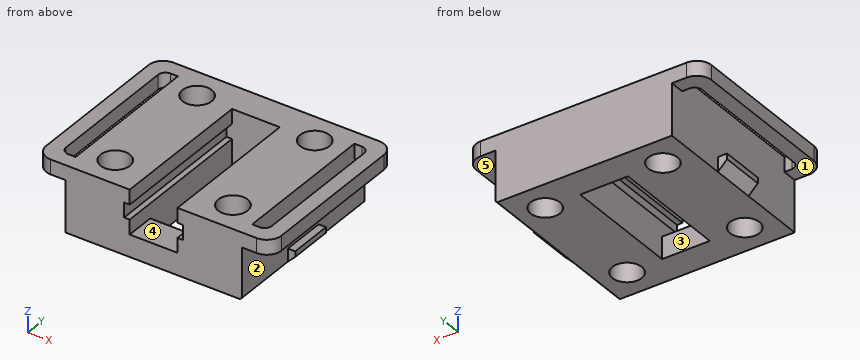
```python
from build123d import *

# Parameters (mm, degrees)
F0_W      = 24
F0_H      = 24
F0_R      = 2
F1_DEPTH  = 9
F3_START  = 7
F2_W      = 32
F2_H      = 24
F2_R      = 2
F2_W_2    = 2
F2_H_2    = 20
F3_DEPTH  = 2
F4_W      = 8
F4_H      = 6
F5_DEPTH  = 12
F6_DEPTH  = 8
F7_W      = 0.75
F7_H      = 2
F8_DEPTH  = 12
F9_W      = 1.25
F9_H      = 6
F10_DEPTH = 2
F11_SIZE  = 1.25
F12_W     = 6.5
F12_H     = 16
F13_DEPTH = 3
F14_R     = 2
F15_R     = 1


with BuildPart() as f1:
    # F0 (on Top) → F1 (new body)
    with BuildSketch(Plane.XY):
        Rectangle(F0_W, F0_H)
        with Locations((-8, -8)):
            Circle(F0_R, mode=Mode.SUBTRACT)
        with Locations((8, -8)):
            Circle(F0_R, mode=Mode.SUBTRACT)
        with Locations((-8, 8)):
            Circle(F0_R, mode=Mode.SUBTRACT)
        with Locations((8, 8)):
            Circle(F0_R, mode=Mode.SUBTRACT)
    extrude(amount=F1_DEPTH)

    # F2 (on Top) → F3 (join)
    with BuildSketch(Plane.XY.offset(F3_START)):
        Rectangle(F2_W, F2_H)
        with Locations((-8, -8)):
            Circle(F2_R, mode=Mode.SUBTRACT)
        with Locations((8, -8)):
            Circle(F2_R, mode=Mode.SUBTRACT)
        with Locations((-13, 0)):
            Rectangle(F2_W_2, F2_H_2, mode=Mode.SUBTRACT)
        with Locations((-8, 8)):
            Circle(F2_R, mode=Mode.SUBTRACT)
        with Locations((13, 0)):
            Rectangle(F2_W_2, F2_H_2, mode=Mode.SUBTRACT)
        with Locations((8, 8)):
            Circle(F2_R, mode=Mode.SUBTRACT)
    extrude(amount=F3_DEPTH)

    # F4 (on Front) → F5 (cut)
    with BuildSketch(Plane.XZ):
        with Locations((0, 6)):
            Rectangle(F4_W, F4_H)
    extrude(amount=F5_DEPTH, mode=Mode.SUBTRACT)

    # F4 (on Front) → F6 (cut)
    with BuildSketch(Plane.XZ):
        with Locations((0, 6)):
            Rectangle(F4_W, F4_H)
    extrude(amount=-F6_DEPTH, mode=Mode.SUBTRACT)

    # F7 (on Front) → F8 (join, symmetric)
    with BuildSketch(Plane.XZ):
        with Locations((-3.625, 8)):
            Rectangle(F7_W, F7_H)
        with Locations((3.625, 8)):
            Rectangle(F7_W, F7_H)
        with Locations((3.625, 4)):
            Rectangle(F7_W, F7_H)
        with Locations((-3.625, 4)):
            Rectangle(F7_W, F7_H)
    extrude(amount=F8_DEPTH, both=True)

    # F9 (on Top) → F10 (join)
    with BuildSketch(Plane.XY):
        with Locations((-12.625, 0)):
            Rectangle(F9_W, F9_H)
        with Locations((12.375, 0)):
            Rectangle(F9_W, F9_H)
    extrude(amount=F10_DEPTH)

    # F11
    f11_edges = [f1.edges().sort_by_distance(p)[0] for p in [
        (13, 0, 0),
        (-13.25, 0, 0),
    ]]
    chamfer(f11_edges, length=F11_SIZE)

    # F12 (on Top) → F13 (cut)
    with BuildSketch(Plane.XY):
        Rectangle(F12_W, F12_H)
    extrude(amount=F13_DEPTH, mode=Mode.SUBTRACT)

    # F14
    f14_edges = [f1.edges().sort_by_distance(p)[0] for p in [
        (16, -12, 8),
        (16, 12, 8),
        (-16, -12, 8),
        (-16, 12, 8),
    ]]
    fillet(f14_edges, radius=F14_R)

    # F15
    f15_edges = [f1.edges().sort_by_distance(p)[0] for p in [
        (-14, 10, 8),
        (-14, -10, 8),
        (14, 10, 8),
        (14, -10, 8),
    ]]
    fillet(f15_edges, radius=F15_R)


solid = f1.part
```
Check sheet for the modelled part. Datum: model origin and axes. Units: mm. Face numbers are marked on the shaded views. A direction names the side the tool comes from. Give positions to 0.01 mm unless a question says otherwise; leave off trailing zeros. Order: outer loops, then holes, each group sorted by start corner. A loop starts at its lowest first (then second) coordinate and runs counter-clockwise, first axis right, second up. Notation, with made-up numbers: (64.5, -13.75) -> (68.5, -13.75) arc R22 cw to (68.5, 10.25) -> close; hole circle Ø7 at (17.25, 28.5). An arc over 180 degrees is marked (long way). Use CSV: the item, a comma, the result in double quotes. Start each with the question number.
1) Sectioned sample at A-A, the plane x = -8. Record the boundary of the cut face in (y, z), plus the area to 3 significant figures.
2) Sectioned sample at C-C, the plane x = 1.5. Record the boundary of the cut face in (y, z).
3) Sectioned sample at D-D, the plane z = 6.5. Record the boundary of the cut face in (x, y).
4) Set-up check for the marked faces 3, 4 and 5: record each of +Z, -Z, +X, -X, +Y, -Y from which the full face is reachable in a straight line by a thin tool's end or side.
5) Material ranges on line 1 (Y direction, x = -8, z = 6.25); line 2 (X direction, y = 4.75, z = 7.5); line 3 (X direction, y = -2, z = 4), recorded low to high. Write a range as from..to.
6) Go/stop test with flat-tipped pins: P1, Ø4, axis at x = -1.5, z = 4.5, coming from the -Y side; P2, Ø0.6, axis at y = 2, z = 6, coming from the +X side; P3, Ø4.5, axis at y = 2.5, z = 3.5, coming from the -X side; P4, Ø1, axis at y = -0.5, z = 6, coming from the -X side. Record where each tip stops, or that it passes through.
7) Mould release check, pull along X, two halves, no side actions. Record for the marked faces 1 and 2: released by +X, released by -X, zero draft, split by the parting line, or undercut.
8) Sectioned sample at B-B, the plane y = -0.25. Give the number of separate pieces and of enclosed holes in the cut face, plus the area to 3 significant figures.
Recorded:
1,outline,"(-12, 0) -> (-10, 0) -> (-10, 9) -> (-12, 9) -> close; (-6, 0) -> (6, 0) -> (6, 9) -> (-6, 9) -> close; (10, 0) -> (12, 0) -> (12, 9) -> (10, 9) -> close"
1,area,"144 mm2"
2,outline,"(-12, 0) -> (-8, 0) -> (-8, 3) -> (-12, 3) -> close; (8, 0) -> (12, 0) -> (12, 9) -> (8, 9) -> close"
3,outline,"(-12, -12) -> (-4, -12) -> (-4, 8) -> (4, 8) -> (4, -12) -> (12, -12) -> (12, 12) -> (-12, 12) -> close; hole circle Ø4 at (-8, -8); hole circle Ø4 at (-8, 8); hole circle Ø4 at (8, -8); hole circle Ø4 at (8, 8)"
4,face 3,"+Z, -Z"
4,face 4,"+Z, -Y"
4,face 5,"-Z, +X, +Y, -Y"
5,line 1,"-12..-10, -6..6, 10..12"
5,line 2,"-16..-14, -12..-3.25, 3.25..12, 14..16"
5,line 3,"-12..-3.25, 3.25..12"
6,P1,"y = -12"
6,P2,"x = 12"
6,P3,"x = -13.25"
6,P4,"x = -12"
7,face 1,"zero draft"
7,face 2,"undercut"
8,separate pieces,"4"
8,enclosed holes,"0"
8,area,"165 mm2"
